Verification items for the finished model (mm, model axes). Face numbers are marked on the shaded views. Coordinates: 2 decimals unless noted, no trailing zeros. Write each loop counter-clockwise with the first axis right and the second up, starting at its lowest first coordinate (ties: lowest second). Pieces come first, ordered by that corner, then holes. Notation, with made-up numbers: (-21.75, -33.75) - (23.25, -33.75) arc R14 ccw to (23.25, -26.75) - close; hole circle Ø1 at (-33.75, -13.5). An arc over 180 degrees is marked (long way). Answer as CSV lines item,"result". Start each with the question number.
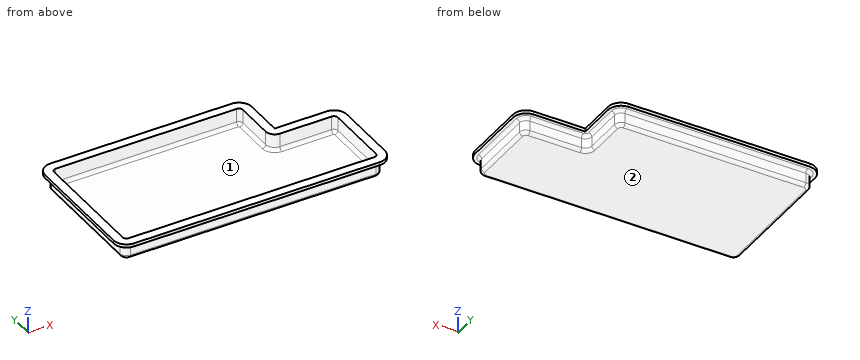
```python
from build123d import *

# Parameters (mm, degrees)
F1_DEPTH = 30
F2_T     = -4
F4_DEPTH = 5
F5_R     = 5
F6_R     = 5


with BuildPart() as f1:
    # F0 (on Top) → F1 (new body)
    with BuildSketch(Plane.XY):
        with BuildLine():
            ThreePointArc((-83.0841619524, 140.1000192761), (-90.1552297642, 137.171087088), (-93.0841619524, 130.1000192761))
            Line((-93.0841619524, 130.1000192761), (-93.0841619524, -49.8999807239))
            ThreePointArc((-93.0841619524, -49.8999807239), (-90.1552297642, -56.9710485357), (-83.0841619524, -59.8999807239))
            Line((-83.0841619524, -59.8999807239), (296.9158380476, -59.8999807239))
            ThreePointArc((296.9158380476, -59.8999807239), (303.9869058595, -56.9710485357), (306.9158380476, -49.8999807239))
            Line((306.9158380476, -49.8999807239), (306.9158380476, 50.1000192761))
            ThreePointArc((306.9158380476, 50.1000192761), (303.9869058595, 57.171087088), (296.9158380476, 60.1000192761))
            Line((296.9158380476, 60.1000192761), (216.9158380476, 60.1000192761))
            ThreePointArc((216.9158380476, 60.1000192761), (209.8447702358, 63.0289514643), (206.9158380476, 70.1000192761))
            Line((206.9158380476, 70.1000192761), (206.9158380476, 130.1000192761))
            ThreePointArc((206.9158380476, 130.1000192761), (203.9869058595, 137.171087088), (196.9158380476, 140.1000192761))
            Line((196.9158380476, 140.1000192761), (-83.0841619524, 140.1000192761))
        make_face()
    extrude(amount=F1_DEPTH)

    # F2
    f2_openings = [f1.faces().sort_by_distance(p)[0] for p in [
        (90.23061, 33.426728, 30),
    ]]
    offset(amount=F2_T, openings=f2_openings)

    # F3 (on face) → F4 (join)
    with BuildSketch(Plane.XY.offset(30)):
        with BuildLine():
            Line((196.9158380476, 150.1000192761), (-83.0841619524, 150.1000192761))
            ThreePointArc((-83.0841619524, 150.1000192761), (-97.2262975761, 144.2421548999), (-103.0841619524, 130.1000192761))
            Line((-103.0841619524, 130.1000192761), (-103.0841619524, -49.8999807239))
            ThreePointArc((-103.0841619524, -49.8999807239), (-97.2262975761, -64.0421163476), (-83.0841619524, -69.8999807239))
            Line((-83.0841619524, -69.8999807239), (296.9158380476, -69.8999807239))
            ThreePointArc((296.9158380476, -69.8999807239), (311.0579736714, -64.0421163476), (316.9158380476, -49.8999807239))
            Line((316.9158380476, -49.8999807239), (316.9158380476, 50.1000192761))
            ThreePointArc((316.9158380476, 50.1000192761), (311.0579736714, 64.2421548999), (296.9158380476, 70.1000192761))
            Line((296.9158380476, 70.1000192761), (216.9158380476, 70.1000192761))
            Line((216.9158380476, 70.1000192761), (216.9158380476, 130.1000192761))
            ThreePointArc((216.9158380476, 130.1000192761), (211.0579736714, 144.2421548999), (196.9158380476, 150.1000192761))
        make_face()
        with BuildLine():
            ThreePointArc((196.9158380476, 136.1000192761), (201.1584787347, 134.3426599633), (202.9158380476, 130.1000192761))
            Line((202.9158380476, 130.1000192761), (202.9158380476, 70.1000192761))
            ThreePointArc((202.9158380476, 70.1000192761), (207.016343111, 60.2005243395), (216.9158380476, 56.1000192761))
            Line((216.9158380476, 56.1000192761), (296.9158380476, 56.1000192761))
            ThreePointArc((296.9158380476, 56.1000192761), (301.1584787347, 54.3426599633), (302.9158380476, 50.1000192761))
            Line((302.9158380476, 50.1000192761), (302.9158380476, -49.8999807239))
            ThreePointArc((302.9158380476, -49.8999807239), (301.1584787347, -54.142621411), (296.9158380476, -55.8999807239))
            Line((296.9158380476, -55.8999807239), (-83.0841619524, -55.8999807239))
            ThreePointArc((-83.0841619524, -55.8999807239), (-87.3268026395, -54.142621411), (-89.0841619524, -49.8999807239))
            Line((-89.0841619524, -49.8999807239), (-89.0841619524, 130.1000192761))
            ThreePointArc((-89.0841619524, 130.1000192761), (-87.3268026395, 134.3426599633), (-83.0841619524, 136.1000192761))
            Line((-83.0841619524, 136.1000192761), (196.9158380476, 136.1000192761))
        make_face(mode=Mode.SUBTRACT)
    extrude(amount=-F4_DEPTH)

    # F5
    f5_edges = [f1.edges().sort_by_distance(p)[0] for p in [
        (256.915838, 56.100019, 4),
        (207.016343, 60.200524, 4),
        (202.915838, 100.100019, 4),
        (201.158479, 134.34266, 4),
        (56.915838, 136.100019, 4),
        (-87.326803, 134.34266, 4),
        (-89.084162, 40.100019, 4),
        (-87.326803, -54.142621, 4),
        (106.915838, -55.899981, 4),
        (301.158479, -54.142621, 4),
        (302.915838, 0.100019, 4),
        (301.158479, 54.34266, 4),
    ]]
    fillet(f5_edges, radius=F5_R)

    # F6
    f6_edges = [f1.edges().sort_by_distance(p)[0] for p in [
        (106.915838, -59.899981, 25),
        (106.915838, -59.899981, 0),
    ]]
    fillet(f6_edges, radius=F6_R)


solid = f1.part
```
1. Scan lines: line 1 along Y through (x, z) = (252.5, 12.5); line 2 along X through (y, z) = (84.5, 27.5); line 3 along X through (y, z) = (34.5, 18.5). Record each from-to range of solid material in increasing order. Write a range as from..to.
2. Cross-section at B-B (x = -60). Record the cut outline in (y, z).
3. Depth check by flat-ended pin: P1, Ø5, axis at y = -36.5, z = 23, coming from the +X side; P2, Ø1.5, axis at x = 198, z = 24.5, coming from the +Y side; P3, Ø1.5, axis at y = 20, z = 13, coming from the +X side; P4, Ø1, axis at x = 87.5, y = 64, coming from the +Z side. Enter the tip coordinate at first touch or a pass-through.
4. Cross-section at A-A (y = -22.5). Record the cut outline in (x, z).
5. Draft check along Y on the marked faces 1 and 2. Enter one of: pulls with the +Y half, pulls with the -Y half, needs draft (parallel to the pull), parting line crosses it, or undercut.
Completed:
1,line 1,"y = -59.9..-55.9, 56.1..60.1"
1,line 2,"x = -103.08..-89.08, 202.92..216.92"
1,line 3,"x = -93.08..-89.08, 302.92..306.92"
2,outline,"(-69.9, 25) - (-64.9, 25) arc R5 cw to (-59.9, 20) - (-59.9, 5) arc R5 ccw to (-54.9, 0) - (135.1, 0) arc R5 ccw to (140.1, 5) - (140.1, 20) arc R5 cw to (145.1, 25) - (150.1, 25) - (150.1, 30) - (136.1, 30) - (136.1, 9) arc R5 cw to (131.1, 4) - (-50.9, 4) arc R5 cw to (-55.9, 9) - (-55.9, 30) - (-69.9, 30) - close"
3,P1,"stops at x = 316.92"
3,P2,"stops at y = 150.09"
3,P3,"stops at x = 306.92"
3,P4,"stops at z = 4"
4,outline,"(-103.08, 25) - (-98.08, 25) arc R5 cw to (-93.08, 20) - (-93.08, 5) arc R5 ccw to (-88.08, 0) - (301.92, 0) arc R5 ccw to (306.92, 5) - (306.92, 20) arc R5 cw to (311.92, 25) - (316.92, 25) - (316.92, 30) - (302.92, 30) - (302.92, 9) arc R5 cw to (297.92, 4) - (-84.08, 4) arc R5 cw to (-89.08, 9) - (-89.08, 30) - (-103.08, 30) - close"
5,face 1,"undercut"
5,face 2,"needs draft"
